Design review of the part built by this model. Coordinates are the model's own, in mm. A direction names the side the tool comes from. Round coordinates to 2 decimals unless told otherwise and drop trailing zeros. Loops run counter-clockwise (first coordinate to the right, second up) from the corner with the lowest first, then second, coordinate; pieces in that order, holes last. Notation, with made-up numbers: (43, -9) -> (70, -9) arc R28 ccw to (70, 18) -> close; hole circle Ø2 at (10.25, 28). An arc over 180 degrees is marked (long way). Answer as CSV lines item,"result". Start each with the question number.
(1) Draft analysis for pull direction Z (two halves, no side actions). For faces 1 (the face through (4.436, 13.804, -2.307)), 2 (the face through (-1.802, 22.93, -5.723)), 3 (the face through (-4, 28, 4)), state which applies: +Z half, -Z half, draft (parallel to the pull), parting line (faces both ways), or undercut.
(2) Take a section at C-C, the plane z = 17. Write out the cut boundary in (x, y).
(3) Take a section at B-B, the plane x = -3.5. Write out the cut boundary in (y, z), and give its area (3 significant figures).
(4) Take a section at A-A, the plane z = 0. Write out the cut boundary in (x, y), and give its area (3 significant figures).
(5) Machinability: for faces 4 (the face through (-1.802, 5.07, -5.723)), 5 (the face through (0, 16, -13)), which of the approach directions +Z, -Z, +X, -X, +Y, -Y give a long, thin tool a straight path to every point of the face, cutting with its end or side? Answer none if there is none.
(6) For P1, Ø1, axis at y = 7.5, z = -1.5, coming from the -X side; P2, Ø8, axis at y = 4.5, z = 6, coming from the +X side; P3, Ø3, axis at x = -7, y = 24, coming from the -Z side, all flat-tipped, find the tip position at first contact; note any pin that passes through.
(7) Take a section at D-D, the plane y = 19.75. Write out the cut boundary in (x, z), and give its area (3 significant figures).
(8) To check wall thickness, follow line 1 (Y direction, x = 0, z = 5.1); line 2 (X direction, y = 9.5, z = 0); line 3 (X direction, y = 14, z = 13.5). State the ranges of each line that lie inside material, in increasing order. Write a range as from..to.
from build123d import *

# Parameters (mm, degrees)
SKETCH2_R               = 6
SKETCH2_R_2             = 5
BOSS_EXTRUDE1_DEPTH     = 10
SKETCH3_R               = 1.5
CUT_EXTRUDE1_DEPTH      = 46.299006612
CUT_EXTRUDE2_DEPTH      = 42.85689914
CUT_EXTRUDE2_DEPTH_BACK = 42.85689914
SKETCH4_R               = 2
SKETCH5_W               = 20
SKETCH5_H               = 45
CUT_EXTRUDE3_DEPTH      = 10


with BuildPart() as part:
    # Sketch1 → Revolve1 (revolve)
    with BuildSketch(Plane.XY, mode=Mode.PRIVATE) as revolve1_sk:
        Polygon((5, 0), (6, 0), (6, 10), (22, 10), (22, 18), (5, 18), (5, 13), align=None)
    revolve(revolve1_sk.sketch.rotate(Axis((0, 0, 0), (0, 1, 0)), 90), axis=Axis((0, 0, 0), (0, 1, 0)))

    # Sketch2 → Boss-Extrude1 (add)
    with BuildSketch(Plane(origin=(0, 18, 0), x_dir=(1, 0, 0), z_dir=(0, 1, 0))):
        with Locations(Location((0, 0, 0), (0, 0, 90))):
            Circle(SKETCH2_R)
        with Locations(Location((0, 0, 0), (0, 0, 90))):
            Circle(SKETCH2_R_2, mode=Mode.SUBTRACT)
    extrude(amount=BOSS_EXTRUDE1_DEPTH)

    # Sketch3 → Cut-Extrude1 (cut, through all)
    with BuildSketch(Plane(origin=(0, 0, -6), x_dir=(-1, 0, 0), z_dir=(0, 0, -1))):
        with Locations((0, 5)):
            Circle(SKETCH3_R)
        with Locations((0, 23)):
            Circle(SKETCH3_R)
    extrude(amount=-CUT_EXTRUDE1_DEPTH, mode=Mode.SUBTRACT)

    # Sketch4 → Cut-Extrude2 (cut, two sides: drawn at the far end of the back side and taken through both)
    with BuildSketch(Plane.XY.offset(-CUT_EXTRUDE2_DEPTH_BACK)):
        with Locations((0, 14)):
            Circle(SKETCH4_R)
    extrude(amount=CUT_EXTRUDE2_DEPTH + CUT_EXTRUDE2_DEPTH_BACK, mode=Mode.SUBTRACT)

    # Sketch5 → Cut-Extrude3 (cut)
    with BuildSketch(Plane.XZ.offset(-10)):
        with Locations((-20, 0)):
            Rectangle(SKETCH5_W, SKETCH5_H)
        with Locations((20, 0)):
            Rectangle(SKETCH5_W, SKETCH5_H)
    extrude(amount=-CUT_EXTRUDE3_DEPTH, mode=Mode.SUBTRACT)


solid = part.part
The answers:
1,face 1,"undercut"
1,face 2,"parting line"
1,face 3,"draft"
2,outline,"(-10, 10) -> (10, 10) -> (10, 18) -> (-10, 18) -> close; hole circle Ø4 at (0, 14)"
3,outline,"(0, -4.87) -> (10, -4.87) -> (10, -21.72) -> (18, -21.72) -> (18, -4.87) -> (28, -4.87) -> (28, -3.57) -> (0, -3.57) -> close; (0, 3.57) -> (28, 3.57) -> (28, 4.87) -> (18, 4.87) -> (18, 21.72) -> (10, 21.72) -> (10, 4.87) -> (0, 4.87) -> close"
3,area,"342 mm²"
4,outline,"(-10, 10) -> (-6, 10) -> (-6, 0) -> (-5, 0) -> (-5, 28) -> (-6, 28) -> (-6, 18) -> (-10, 18) -> close; (5, 0) -> (6, 0) -> (6, 10) -> (10, 10) -> (10, 18) -> (6, 18) -> (6, 28) -> (5, 28) -> close"
4,area,"120 mm²"
5,face 4,"-Y"
5,face 5,"+Z, -Z"
6,P1,"x = -5.92"
6,P2,"x = 5.66"
6,P3,"z = -2.4"
7,outline,"circle Ø12 at (0, 0); hole circle Ø10 at (0, 0)"
7,area,"34.6 mm²"
8,line 1,"0..3.5, 6.5..12, 16..21.5, 24.5..28"
8,line 2,"-6..-5, 5..6"
8,line 3,"-10..-2, 2..10"
